```python
from build123d import *

# Parameters (mm, degrees)
SKETCH1_W           = 7.9375
SKETCH1_H           = 9.525
EXTRUDE1_DEPTH      = 3.96875
SKETCH2_OUTSIDE_W   = 12.541
SKETCH2_OUTSIDE_H   = 8.573
EXTRUDE2_DEPTH      = 14.018467952
EXTRUDE3_DEPTH      = 1.5875
EXTRUDE4_DEPTH      = 6.35
BOSS_EXTRUDE1_START = -2.54
BOSS_EXTRUDE1_DEPTH = 1.2192


with BuildPart() as part:
    # Sketch1 → Extrude1 (new body)
    with BuildSketch(Plane(origin=(0, 0, 0), x_dir=(1, 0, 0), z_dir=(0, 1, 0))):
        with Locations((3.96875, 4.7625)):
            Rectangle(SKETCH1_W, SKETCH1_H)
    extrude(amount=EXTRUDE1_DEPTH)

    # Sketch2 outside → Extrude2 (cut, through all)
    with BuildSketch(Plane.XY):
        with Locations((3.9685, 1.9845)):
            Rectangle(SKETCH2_OUTSIDE_W, SKETCH2_OUTSIDE_H)
        with BuildLine():
            Line((0, 1.984375), (0, 3.571875))
            ThreePointArc((0, 3.571875), (0.116241996, 3.852508004), (0.396875, 3.96875))
            Line((0.396875, 3.96875), (7.540625, 3.96875))
            ThreePointArc((7.540625, 3.96875), (7.821258004, 3.852508004), (7.9375, 3.571875))
            Line((7.9375, 3.571875), (7.9375, 1.984375))
            ThreePointArc((7.9375, 1.984375), (7.821258004, 1.703741996), (7.540625, 1.5875))
            Line((7.540625, 1.5875), (7.3421875, 1.5875))
            ThreePointArc((7.3421875, 1.5875), (7.061554496, 1.471258004), (6.9453125, 1.190625))
            Line((6.9453125, 1.190625), (6.9453125, 0.396875))
            ThreePointArc((6.9453125, 0.396875), (6.829070504, 0.116241996), (6.5484375, 0))
            Line((6.5484375, 0), (1.3890625, 0))
            ThreePointArc((1.3890625, 0), (1.108429496, 0.116241996), (0.9921875, 0.396875))
            Line((0.9921875, 0.396875), (0.9921875, 1.190625))
            ThreePointArc((0.9921875, 1.190625), (0.875945504, 1.471258004), (0.5953125, 1.5875))
            Line((0.5953125, 1.5875), (0.396875, 1.5875))
            ThreePointArc((0.396875, 1.5875), (0.116241996, 1.703741996), (0, 1.984375))
        make_face(mode=Mode.SUBTRACT)
    extrude(amount=-EXTRUDE2_DEPTH, mode=Mode.SUBTRACT)

    # Sketch3 → Extrude3 (cut)
    with BuildSketch(Plane.XY):
        with BuildLine():
            ThreePointArc((1.3890625, 1.190625), (1.156578508, 1.751891008), (0.5953125, 1.984375))
            Line((0.5953125, 1.984375), (0.49609375, 1.984375))
            ThreePointArc((0.49609375, 1.984375), (0.425935499, 2.013435499), (0.396875, 2.08359375))
            Line((0.396875, 2.08359375), (0.396875, 3.175))
            ThreePointArc((0.396875, 3.175), (0.513116996, 3.455633004), (0.79375, 3.571875))
            Line((0.79375, 3.571875), (7.14375, 3.571875))
            ThreePointArc((7.14375, 3.571875), (7.424383004, 3.455633004), (7.540625, 3.175))
            Line((7.540625, 3.175), (7.540625, 2.08359375))
            ThreePointArc((7.540625, 2.08359375), (7.511564501, 2.013435499), (7.44140625, 1.984375))
            Line((7.44140625, 1.984375), (7.3421875, 1.984375))
            ThreePointArc((7.3421875, 1.984375), (6.780921492, 1.751891008), (6.5484375, 1.190625))
            Line((6.5484375, 1.190625), (6.5484375, 0.396875))
            Line((6.5484375, 0.396875), (1.3890625, 0.396875))
            Line((1.3890625, 0.396875), (1.3890625, 1.190625))
        make_face()
    extrude(amount=-EXTRUDE3_DEPTH, mode=Mode.SUBTRACT)

    # Sketch5 → Extrude4 (cut)
    with BuildSketch(Plane.XY.offset(-1.5875)):
        with BuildLine():
            Line((0.79375, 3.571875), (7.14375, 3.571875))
            ThreePointArc((7.14375, 3.571875), (7.424383004, 3.455633004), (7.540625, 3.175))
            Line((7.540625, 3.175), (7.540625, 2.08359375))
            ThreePointArc((7.540625, 2.08359375), (7.511564501, 2.013435499), (7.44140625, 1.984375))
            Line((7.44140625, 1.984375), (7.3421875, 1.984375))
            ThreePointArc((7.3421875, 1.984375), (6.780921492, 1.751891008), (6.5484375, 1.190625))
            Line((6.5484375, 1.190625), (6.5484375, 0.396875))
            Line((6.5484375, 0.396875), (1.3890625, 0.396875))
            Line((1.3890625, 0.396875), (1.3890625, 1.190625))
            ThreePointArc((1.3890625, 1.190625), (1.156578508, 1.751891008), (0.5953125, 1.984375))
            Line((0.5953125, 1.984375), (0.49609375, 1.984375))
            ThreePointArc((0.49609375, 1.984375), (0.425935499, 2.013435499), (0.396875, 2.08359375))
            Line((0.396875, 2.08359375), (0.396875, 3.175))
            ThreePointArc((0.396875, 3.175), (0.513116996, 3.455633004), (0.79375, 3.571875))
        make_face()
        with BuildLine():
            Line((1.824986809, 2.778125), (6.219655485, 2.778125))
            ThreePointArc((6.219655485, 2.778125), (6.29171032, 2.545641008), (6.219655485, 2.313157015))
            Line((6.219655485, 2.313157015), (5.805428146, 1.313123756))
            ThreePointArc((5.805428146, 1.313123756), (5.73234177, 1.224067749), (5.622095802, 1.190625))
            Line((5.622095802, 1.190625), (2.315404198, 1.190625))
            ThreePointArc((2.315404198, 1.190625), (2.20515823, 1.224067749), (2.132071854, 1.313123756))
            Line((2.132071854, 1.313123756), (1.717844515, 2.313157015))
            ThreePointArc((1.717844515, 2.313157015), (1.697050338, 2.562776965), (1.824986809, 2.778125))
        make_face(mode=Mode.SUBTRACT)
    extrude(amount=-EXTRUDE4_DEPTH, mode=Mode.SUBTRACT)

    # Sketch6 → Boss-Extrude1 (add)
    with BuildSketch(Plane.XY.offset(BOSS_EXTRUDE1_START)):
        with BuildLine():
            Line((0, 3.139540901), (0, 0.523875))
            ThreePointArc((0, 0.523875), (-0.037197439, 0.434072439), (-0.127, 0.396875))
            Line((-0.127, 0.396875), (-0.523875, 0.396875))
            ThreePointArc((-0.523875, 0.396875), (-0.613677561, 0.359677561), (-0.650875, 0.269875))
            Line((-0.650875, 0.269875), (-0.650875, 0.127))
            ThreePointArc((-0.650875, 0.127), (-0.613677561, 0.037197439), (-0.523875, 0))
            Line((-0.523875, 0), (0.269875, 0))
            ThreePointArc((0.269875, 0), (0.359677561, 0.037197439), (0.396875, 0.127))
            Line((0.396875, 0.127), (0.396875, 3.139540901))
            Line((0.396875, 3.139540901), (0, 3.139540901))
        make_face()
        with BuildLine():
            Line((7.540625, 3.139540901), (7.9375, 3.139540901))
            Line((7.9375, 3.139540901), (7.9375, 0.523875))
            ThreePointArc((7.9375, 0.523875), (7.974697439, 0.434072439), (8.0645, 0.396875))
            Line((8.0645, 0.396875), (8.461375, 0.396875))
            ThreePointArc((8.461375, 0.396875), (8.551177561, 0.359677561), (8.588375, 0.269875))
            Line((8.588375, 0.269875), (8.588375, 0.127))
            ThreePointArc((8.588375, 0.127), (8.551177561, 0.037197439), (8.461375, 0))
            Line((8.461375, 0), (7.667625, 0))
            ThreePointArc((7.667625, 0), (7.577822439, 0.037197439), (7.540625, 0.127))
            Line((7.540625, 0.127), (7.540625, 3.139540901))
        make_face()
    extrude(amount=-BOSS_EXTRUDE1_DEPTH)


solid = part.part
```
Here's how the part is built. I have some questions about the finished solid (model axes, mm). A direction names the side the tool comes from. Round coordinates to 2 decimals unless told otherwise and drop trailing zeros.
1. For faces 4 (the face through (0.2, 0.6, -2.54)), 5 (the face through (4, 0.397, -4)), 6 (the face through (7.938, 2.4, -4.7)), 7 (the face through (0.397, 1, -3)), which set-ups out of +Z, -Z, +X, -X, +Y, -Y let a thin tool reach every point of the face, with its end or its side?
Answers:
face 4: +Z, -X, -Y
face 5: +Z
face 6: +Z, -Z, +X, +Y
face 7: +Z, -Z, -Y
2. Suppose I cut it at A-A, the plane y = 0.7. Give the number of separate pieces and of enclosed holes in the cut face, and give its area (3 significant figures).
Answers:
separate pieces: 3
enclosed holes: 0
area: 16.7 mm2
3. Will these pins go through, and if not, where does the flat tip stop? pin 1 (0.5 mm diameter, centred on y = 2.5, z = -4.5, fed in from +X); pin 2 (1.3 mm diameter, centred on x = 4, y = 2.5, fed in from +Z); pin 3 (0.9 mm diameter, centred on y = 1, z = -3.5, fed in from -X).
Answers:
pin 1: stops at x = 7.94
pin 2: stops at z = -1.59
pin 3: stops at x = 0
4. Thinking about a two-plate mould opening in X: for faces 1 (the face through (0.2, 0.6, -3.759)), 2 (the face through (0, 2.4, -4.7)), 3 (the face through (4, 2, -1.588)), which applies, released by +X, released by -X, zero draft, split by the parting line, or undercut?
Answers:
face 1: zero draft
face 2: released by -X
face 3: undercut
5. If I drill on probe 1 along Y at (x, z) = (3.75, -5); probe 2 along X at (y, z) = (2.6, -5.25); probe 3 along X at (y, z) = (1.7, -7.75), over which ranges is the centre line in solid material (lowest first)?
Answers:
probe 1: y = 0 to 0.4, 1.19 to 2.78, 3.57 to 3.97
probe 2: x = 0 to 0.4, 1.71 to 6.29, 7.54 to 7.94
probe 3: x = 0.12 to 1.2, 1.97 to 5.97, 6.73 to 7.82
